Input: part model. Units: mm. Frame: model coordinates. A direction names the side the tool comes from. Coordinates: 2 decimals unless noted, no trailing zeros. Order: outer loops, then holes, each group sorted by start corner. A loop starts at its lowest first (then second) coordinate and runs counter-clockwise, first axis right, second up. Notation, with made-up numbers: (-11, -11.5) - (16, -11.5) arc R25 ccw to (16, 12.5) - close; hole circle Ø6 at (88.25, 50.25). An arc over 180 degrees is marked (long way). One line per question, with ' | ' between items.
from build123d import *

# Parameters (mm, degrees)
F0_W     = 25.908
F0_H     = 25.908
F0_R     = 1.778
F1_DEPTH = 3.048
F2_W     = 25.908
F2_H     = 3.048
F3_DEPTH = 28.448
F4_R     = 0.762
F4_R_2   = 1.27
F5_DEPTH = 25.4


with BuildPart() as f1:
    # F0 (on Top) → F1 (new body)
    with BuildSketch(Plane.XY):
        Rectangle(F0_W, F0_H)
        with BuildLine():
            ThreePointArc((-5.1367972132, -6.9147972132), (-8.557455022, -7.595208356), (-5.6575613563, -5.6575613563))
            ThreePointArc((-5.6575613563, -5.6575613563), (-5.2721394044, -6.2343860705), (-5.1367972132, -6.9147972132))
        make_face(mode=Mode.SUBTRACT)
        with Locations((0, -9.779)):
            Circle(F0_R, mode=Mode.SUBTRACT)
        with BuildLine():
            ThreePointArc((8.6927972132, -6.9147972132), (6.2343860705, -8.557455022), (5.6575613563, -5.6575613563))
            ThreePointArc((5.6575613563, -5.6575613563), (7.595208356, -5.2721394044), (8.6927972132, -6.9147972132))
        make_face(mode=Mode.SUBTRACT)
        with Locations((-9.779, 0)):
            Circle(F0_R, mode=Mode.SUBTRACT)
        with BuildLine():
            ThreePointArc((-5.1367972132, 6.9147972132), (-5.2721394044, 6.2343860705), (-5.6575613563, 5.6575613563))
            ThreePointArc((-5.6575613563, 5.6575613563), (-8.557455022, 7.595208356), (-5.1367972132, 6.9147972132))
        make_face(mode=Mode.SUBTRACT)
        with BuildLine():
            ThreePointArc((4.4901280605, 4.4901280605), (5.8666350314, 2.4300397955), (6.35, 0))
            ThreePointArc((6.35, 0), (5.8666350314, -2.4300397955), (4.4901280605, -4.4901280605))
            ThreePointArc((4.4901280605, -4.4901280605), (0, -6.35), (-4.4901280605, -4.4901280605))
            ThreePointArc((-4.4901280605, -4.4901280605), (-6.35, 0), (-4.4901280605, 4.4901280605))
            ThreePointArc((-4.4901280605, 4.4901280605), (0, 6.35), (4.4901280605, 4.4901280605))
        make_face(mode=Mode.SUBTRACT)
        with Locations((9.779, 0)):
            Circle(F0_R, mode=Mode.SUBTRACT)
        with Locations((0, 9.779)):
            Circle(F0_R, mode=Mode.SUBTRACT)
        with BuildLine():
            ThreePointArc((8.6927972132, 6.9147972132), (7.595208356, 5.2721394044), (5.6575613563, 5.6575613563))
            ThreePointArc((5.6575613563, 5.6575613563), (6.2343860705, 8.557455022), (8.6927972132, 6.9147972132))
        make_face(mode=Mode.SUBTRACT)
    extrude(amount=F1_DEPTH)

    # F2 (on face) → F3 (join)
    with BuildSketch(Plane(origin=(0, 0, 0), x_dir=(1, 0, 0), z_dir=(0, 0, -1))):
        with Locations((0, 14.478)):
            Rectangle(F2_W, F2_H)
    extrude(amount=-F3_DEPTH)

    # F4 (on face) → F5 (cut)
    with BuildSketch(Plane.XZ.offset(16.002)):
        with Locations((-8.128, 14.224)):
            Circle(F4_R)
        with Locations((-8.128, 17.78)):
            Circle(F4_R)
        with Locations((-8.128, 10.668)):
            Circle(F4_R)
        with Locations((-3.556, 6.096)):
            Circle(F4_R)
        with Locations((0, 6.096)):
            Circle(F4_R)
        with Locations((3.556, 6.096)):
            Circle(F4_R)
        with Locations((8.128, 10.668)):
            Circle(F4_R)
        with Locations((8.128, 14.224)):
            Circle(F4_R)
        with Locations((8.128, 17.78)):
            Circle(F4_R)
        with Locations((3.556, 22.352)):
            Circle(F4_R)
        with Locations((0, 22.352)):
            Circle(F4_R)
        with Locations((-3.556, 22.352)):
            Circle(F4_R)
        with Locations((0, 14.224)):
            Circle(F4_R_2)
    extrude(amount=-F5_DEPTH, mode=Mode.SUBTRACT)


solid = f1.part
Item 1: Contact query for flat-ended pins moving along their axis: P1, Ø4, axis at y = -12, z = 19, coming from the +X side; P2, Ø4.5, axis at x = -9.779, y = 0, coming from the +Z side; P3, Ø1.5, axis at x = -10, z = 5.5, coming from the +Y side. Output: stop coordinate, or through.
Data:
P1: x = 12.95 | P2: z = 3.05 | P3: y = -12.95
Item 2: Access query for faces 4 (the face through (-3, 6, 3.048)), 5 (the face through (-4.317, -14.499, 6.13)). Directions: +Z, -Z, +X, -X, +Y, -Y. A direction counts if a zero-diameter tool reaches every point of the face in a straight line with its end or side. Return the directions, or none.
Data:
face 4: +Z, +X, -X, +Y | face 5: +Y, -Y
Item 3: Ray query, line 1 (Z direction, x = 0, y = -15.2); line 2 (Z direction, x = -8.5, y = -13.75); line 3 (Z direction, x = -6.75, y = -11.25). Return the intervals inside material, ascending.
Data:
line 1: 0 to 5.33, 6.86 to 12.95, 15.49 to 21.59, 23.11 to 28.45 | line 2: 0 to 10, 11.33 to 13.56, 14.89 to 17.11, 18.45 to 28.45 | line 3: 0 to 3.05
Item 4: Draft query along Y for faces 1 (the face through (0, 12.954, 2)), 2 (the face through (-11.19, -1.08, 1.5)), 3 (the face through (8.029, -14.499, 11.424)). Return one class per face: released by +Y, released by -Y, zero draft, split by the parting line, or undercut.
Data:
face 1: released by +Y | face 2: undercut | face 3: zero draft
Item 5: Section D-D on y = 11. Return the cut outline in (x, z), and give its area (3 significant figures).
Data:
outline: (-12.95, 0) - (-1.29, 0) - (-1.29, 3.05) - (-12.95, 3.05) - close; (1.29, 0) - (12.95, 0) - (12.95, 3.05) - (1.29, 3.05) - close | area: 71.1 mm^2
Item 6: Section C-C on x = 9.75. Return the cut outline in (y, z).
Data:
outline: (-16, 0) - (-1.78, 0) - (-1.78, 3.05) - (-12.95, 3.05) - (-12.95, 28.45) - (-16, 28.45) - close; (1.78, 0) - (12.95, 0) - (12.95, 3.05) - (1.78, 3.05) - close
Item 7: Section A-A on x = 0. Count the separate pieces of the cut face and the enclosed holes in it, and give its area (3 significant figures).
Data:
separate pieces: 7 | enclosed holes: 0 | area: 88.3 mm^2
Item 8: Section B-B on z = 17.78. Return the cut outline in (x, y).
Data:
outline: (-12.95, -16) - (-8.89, -16) - (-8.89, -12.95) - (-12.95, -12.95) - close; (-7.37, -16) - (7.37, -16) - (7.37, -12.95) - (-7.37, -12.95) - close; (8.89, -16) - (12.95, -16) - (12.95, -12.95) - (8.89, -12.95) - close
